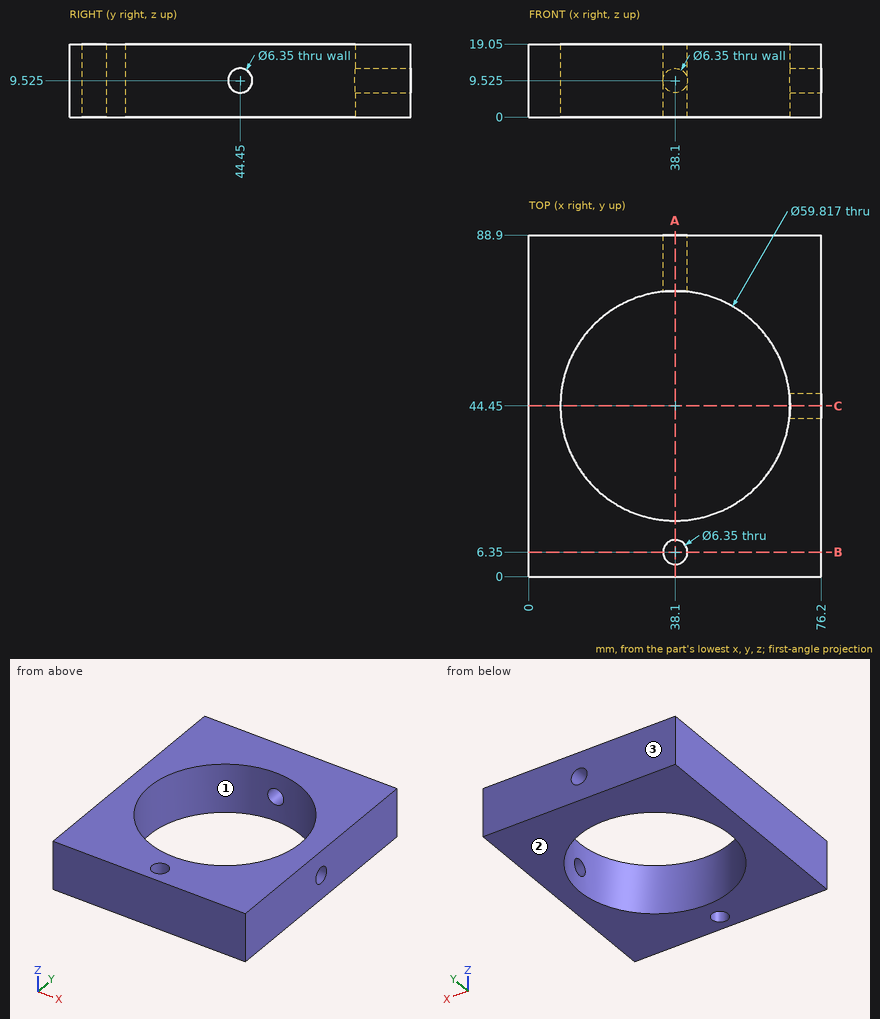
Answer from the drawing. Dimensions are ordinates in mm from the lowest x, y and z of the part. Round coordinates to 2 decimals unless told otherwise and drop trailing zeros. Write each loop counter-clockwise with the first axis right and the second up, starting at its lowest first coordinate (ties: lowest second). Pieces come first, ordered by that corner, then holes. Notation, with made-up numbers: M 62,47 L 109,47 A14 ccw 109,56 Z; hole C 79,-32 d3. An arc over 180 degrees is marked long. Write each question's results on one line, items separated by ' | '. Start each with the question number.
Item 1: A cutting plane is placed at B-B on y = 6.35. Write down the section's boundary in (x, z) (3 decimals).
Item 2: A cutting plane is placed at A-A on x = 38.1. State how many separate pieces and enclosed holes the cut face has, and give its area (3 significant figures).
Item 3: A flat-ended cylindrical pin translates along its axis: pin 1 Ø5.5 at (x, z) = (38.1, 9.525) entering from +Y. Find the tip coordinate at first contact, or state that the pin passes through.
Item 4: A cutting plane is placed at C-C on y = 44.45. Write down the section's boundary in (x, z).
Item 5: For a pull along Y with two mould halves and no side action, classify the marked faces 1, 2 and 3 as pulls with the +Y half, pulls with the -Y half, needs draft (parallel to the pull), parting line crosses it, or undercut.
Item 6: Straight lines are drawn through the part: L1, parallel to Y at x = 38.1, z = 13 (1 decimal); L2, parallel to Z at x = 38.1, y = 79.75; L3, parallel to Y at x = 36.5, z = 4. For each, find the intervals that lie inside material, in ascending order. Write a range as [from, to].
Check sheet entries:
1) outline: M 0,0 L 34.925,0 L 34.925,19.05 L 0,19.05 Z; M 41.275,0 L 76.2,0 L 76.2,19.05 L 41.275,19.05 Z
2) separate pieces: 4 | enclosed holes: 0 | area: 341 mm²
3) pin 1: y = 14.67
4) outline: M 0,0 L 8.19,0 L 8.19,19.05 L 0,19.05 Z; M 68.01,0 L 76.2,0 L 76.2,6.35 L 68.01,6.35 Z; M 68.01,12.7 L 76.2,12.7 L 76.2,19.05 L 68.01,19.05 Z
5) face 1: undercut | face 2: needs draft | face 3: pulls with the +Y half
6) L1: [0, 3.2], [9.5, 14.5], [74.4, 88.9] | L2: [0, 6.35], [12.7, 19.05] | L3: [0, 3.61], [9.09, 14.58], [74.32, 88.9]
